```python
from build123d import *

# Parameters (mm, degrees)
SKETCH2_R           = 12.7
BOSS_EXTRUDE1_DEPTH = 69.85
SKETCH3_R           = 6.45
CUT_EXTRUDE1_DEPTH  = 70.85
CHAMFER1_SIZE       = 2.5


with BuildPart() as part:
    # Sketch2 → Boss-Extrude1 (new body)
    with BuildSketch(Plane.XY):
        Circle(SKETCH2_R)
    extrude(amount=BOSS_EXTRUDE1_DEPTH)

    # Sketch3 → Cut-Extrude1 (cut, through all)
    with BuildSketch(Plane.XY.offset(69.85)):
        Circle(SKETCH3_R)
    extrude(amount=-CUT_EXTRUDE1_DEPTH, mode=Mode.SUBTRACT)

    # Chamfer1
    chamfer1_edges = [part.edges().sort_by_distance(p)[0] for p in [
        (-12.7, 0, 0),
        (-12.7, 0, 69.85),
    ]]
    chamfer(chamfer1_edges, length=CHAMFER1_SIZE)


solid = part.part
```
Here's how the part is built. I have some questions about the finished solid (model axes, mm). Give positions to 0.01 mm unless a question says otherwise; leave off trailing zeros. Write each loop counter-clockwise with the first axis right and the second up, starting at its lowest first coordinate (ties: lowest second). Pieces come first, ordered by that corner, then holes. Notation, with made-up numbers: M -14.75,44.5 L 29.25,44.5 A23 cw 29.25,83.5 Z; hole C 71,-26 d2. An arc over 180 degrees is marked long. Put each result on its own line as item: value. Start each with the question number.
Item 1: Will these pins go through, and if not, where does the flat tip stop? pin 1 (12 mm diameter, centred on x = -1.5, z = 13.5, fed in from -Y); pin 2 (3 mm diameter, centred on y = 9.5, z = 30.5, fed in from -X); pin 3 (7.5 mm diameter, centred on x = 0, y = 0, fed in from +Z); pin 4 (2 mm diameter, centred on y = 3.5, z = 48, fed in from -X).
Item 2: Thinking about a two-plate mould opening in X: for faces 1 (the cylindrical face through (-2.75, -12.4, 34.47)), 2 (the cylindrical face through (-1.398, -6.297, 35.414)), 3 (the flat face through (7, 0, 69.85)), which applies, +X half, -X half, draft (parallel to the pull), parting line (faces both ways), or undercut?
Item 3: I need wall thicknesses on L1, parallel to Y at x = 0, z = 13; L2, parallel to X at y = 0.5, z = 26; L3, parallel to X at y = -3.75, z = 55.5. Which ranges of each line are inside material? Lowest first, please. Write a range as from..to.
Item 4: If we section it at A-A, the plane y = 0: Write out the boundary of the cut face in (x, z).
Item 5: If we section it at C-C, the plane z = 23: Write out the boundary of the cut face in (x, y), then the cut area to 3 significant figures.
Values:
1. pin 1: y = -12.7
1. pin 2: x = -9.86
1. pin 3: through
1. pin 4: x = -12.45
2. face 1: parting line
2. face 2: undercut
2. face 3: draft
3. L1: -12.7..-6.45, 6.45..12.7
3. L2: -12.69..-6.43, 6.43..12.69
3. L3: -12.13..-5.25, 5.25..12.13
4. outline: M -12.7,2.5 L -10.2,0 L -6.45,0 L -6.45,69.85 L -10.2,69.85 L -12.7,67.35 Z; M 6.45,0 L 10.2,0 L 12.7,2.5 L 12.7,67.35 L 10.2,69.85 L 6.45,69.85 Z
5. outline: C 0,0 d25.4; hole C 0,0 d12.9
5. area: 376 mm²
